Autodesk Inventor part; units mm, degrees
ref_plane "YZ Plane" through (0, 0, 0) normal (1, 0, 0) x (0, 1, 0)
ref_plane "XZ Plane" through (0, 0, 0) normal (0, 1, 0) x (-1, 0, 0)
ref_plane "XY Plane" through (0, 0, 0) normal (0, 0, 1) x (1, 0, 0)
sketch "Sketch1" plane through (0, 0, 0) normal (0, 1, 0) x (-1, 0, 0)
  line L0 (0, 0) -> (17, 0)
  line L1 (17, 0) -> (17, -26)
  line L2 (17, -26) -> (0, -26)
  line L3 (0, -26) -> (0, 0)
  dimension "d0" = 26
  dimension "d1" = 17
extrude "Extrusion1" add sketch "Sketch1" along normal blind 46
sketch "Sketch2" plane through (0, 46, 0) normal (0, 1, 0) x (1, 0, 0)
  line L0 (-17, 0) -> (0, 0) construction
  line L1 (-8.5, 0) -> (-8.5, 26) construction
  line L2 (0, 26) -> (-17, 26) construction
  circle A0 centre (-8.5, 20.5) radius 2.8
  line L3 (-3.9389, 6) -> (-6.2195, 2.05)
  line L4 (-6.2195, 2.05) -> (-10.7805, 2.05)
  line L5 (-10.7805, 2.05) -> (-13.0611, 6)
  line L6 (-13.0611, 6) -> (-10.7805, 9.95)
  line L7 (-10.7805, 9.95) -> (-6.2195, 9.95)
  line L8 (-6.2195, 9.95) -> (-3.9389, 6)
  point P0 (-8.5, 6)
  dimension "d5" = 7.9
  dimension "d6" = 6
  dimension "d7" = 5.5
  dimension "d8" = 5.6
extrude "Extrusion2" add sketch "Sketch2" along normal blind 2
equation "\"d2\" = height"
equation "\"height\" = 46"
properties part number "bat9V"
Can you work these out from the model? Positions are in its coordinate system, mm. A direction names the side the tool comes from. Round coordinates to 2 decimals unless told otherwise and drop trailing zeros. Loops run counter-clockwise (first coordinate to the right, second up) from the corner with the lowest first, then second, coordinate; pieces in that order, holes last. Notation, with made-up numbers: (85.5, 80.25) - (104.5, 80.25) arc R30 ccw to (104.5, 116.25) - close; hole circle Ø10 at (37.5, -5.5). An arc over 180 degrees is marked (long way). Answer in a Markdown table with one row per item. Add a question column.
Q1. I want a section at B-B on x = -8.5. List the corners of the cut face in (y, z) for me, and give its area (3 significant figures).
Q2. I need wall thicknesses on L1, parallel to Y at x = -2.75, z = -15. Which ranges of the line are inside material? Lowest first, please.
Q3. We'd pull the mould along Z, two halves only. Please class faces 6 (the flat face through (-8, 47, -2.05)), 7 (the flat face through (-9, 47, -9.95)), 8 (the flat face through (-9, 23, -26)): pulls with the +Z half, pulls with the -Z half, needs draft (parallel to the pull), parting line crosses it, or undercut.
Q4. I want a section at A-A on z = -20.5. List the corners of the cut face in (x, y) for me.
Q5. I want a section at C-C on z = -6.75. List the corners of the cut face in (x, y) for me.
Q6. Which directions (+Z, -Z, +X, -X, +Y, -Y) give clear straight access to the entire face, cutting with the end or side of a thin tool? Please do faces 1 (the flat face through (-8, 46, -13)), 2 (the flat face through (-5.095, 46.986, -8.003)), 3 (the flat face through (-5.063, 46.986, -4.053)), 4 (the flat face through (-11.905, 46.986, -3.997)), 5 (the flat face through (-11.937, 46.986, -7.947)).
Q7. For pin 1 Ø1.6 at (x, y) = (-9, 47) entering from -Z, with a flat end and sliding along its axis, tell me the tip position at first contact or that it passes through.
Q8. I want a section at D-D on x = -2.25. List the corners of the cut face in (y, z) for me.
A:
| question | item | result |
|---|---|---|
| 1 | outline | (0, -26) - (46, -26) - (46, -23.3) - (48, -23.3) - (48, -17.7) - (46, -17.7) - (46, -9.95) - (48, -9.95) - (48, -2.05) - (46, -2.05) - (46, 0) - (0, 0) - close |
| 1 | area | 1,220 mm^2 |
| 2 | L1 | 0 to 46 |
| 3 | face 6 | pulls with the +Z half |
| 3 | face 7 | undercut |
| 3 | face 8 | pulls with the -Z half |
| 4 | outline | (-17, 0) - (0, 0) - (0, 46) - (-5.7, 46) - (-5.7, 48) - (-11.3, 48) - (-11.3, 46) - (-17, 46) - close |
| 5 | outline | (-17, 0) - (0, 0) - (0, 46) - (-4.37, 46) - (-4.37, 48) - (-12.63, 48) - (-12.63, 46) - (-17, 46) - close |
| 6 | face 1 | +Y |
| 6 | face 2 | +X, +Y |
| 6 | face 3 | +Z, +X, +Y |
| 6 | face 4 | +Z, -X, +Y |
| 6 | face 5 | -X, +Y |
| 7 | pin 1 | z = -23.3 |
| 8 | outline | (0, -26) - (46, -26) - (46, 0) - (0, 0) - close |
